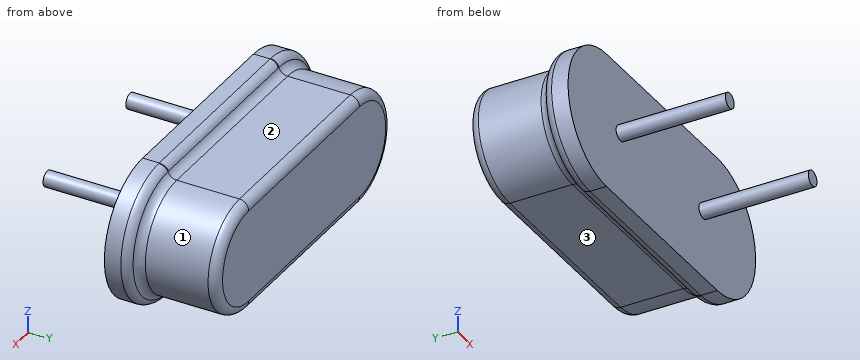
from build123d import *

# Parameters (mm, degrees)
SALIENTE_EXTRUIR1_DEPTH = 3.43
SALIENTE_EXTRUIR2_DEPTH = 0.8
REDONDEO2_R             = 0.3
REDONDEO5_R             = 0.3
CROQUIS2_R              = 0.25
SALIENTE_EXTRUIR3_DEPTH = 3.54


with BuildPart() as part:
    # Croquis1 → Saliente-Extruir1 (new body)
    with BuildSketch(Plane(origin=(0, 0, 0), x_dir=(1, 0, 0), z_dir=(0, 1, 0))):
        with BuildLine():
            Line((0, 0.4), (6.36, 0.4))
            ThreePointArc((6.36, 0.4), (8.16, 2.2), (6.36, 4))
            Line((6.36, 4), (0, 4))
            ThreePointArc((0, 4), (-1.8, 2.2), (0, 0.4))
        make_face()
    extrude(amount=SALIENTE_EXTRUIR1_DEPTH)

    # Croquis1_3 → Saliente-Extruir2 (add)
    with BuildSketch(Plane(origin=(0, 0, 0), x_dir=(1, 0, 0), z_dir=(0, 1, 0))):
        with BuildLine():
            Line((0, 0), (6.36, 0))
            ThreePointArc((6.36, 0), (8.56, 2.2), (6.36, 4.4))
            Line((6.36, 4.4), (0, 4.4))
            ThreePointArc((0, 4.4), (-2.2, 2.2), (0, 0))
        make_face()
        with BuildLine():
            Line((0, 0.4), (6.36, 0.4))
            ThreePointArc((6.36, 0.4), (8.16, 2.2), (6.36, 4))
            Line((6.36, 4), (0, 4))
            ThreePointArc((0, 4), (-1.8, 2.2), (0, 0.4))
        make_face(mode=Mode.SUBTRACT)
    extrude(amount=SALIENTE_EXTRUIR2_DEPTH)

    # Redondeo2
    redondeo2_edges = [part.edges().sort_by_distance(p)[0] for p in [
        (8.16, 3.43, -2.2),
        (3.18, 3.43, -4),
        (-1.8, 0.8, -2.2),
        (3.18, 0.8, -0.4),
        (8.16, 0.8, -2.2),
        (3.18, 0.8, -4),
        (-1.8, 3.43, -2.2),
        (3.18, 3.43, -0.4),
    ]]
    fillet(redondeo2_edges, radius=REDONDEO2_R)

    # Redondeo5
    redondeo5_edges = [part.edges().sort_by_distance(p)[0] for p in [
        (-2.2, 0.8, -2.2),
        (3.18, 0.8, -4.4),
        (8.56, 0.8, -2.2),
        (3.18, 0.8, 0),
    ]]
    fillet(redondeo5_edges, radius=REDONDEO5_R)

    # Croquis2 → Saliente-Extruir3 (add)
    with BuildSketch(Plane.XZ):
        with Locations(Location((0.805, -2.2, 0), (0, 0, 90))):
            Circle(CROQUIS2_R)
        with Locations(Location((5.555, -2.2, 0), (0, 0, 90))):
            Circle(CROQUIS2_R)
    extrude(amount=SALIENTE_EXTRUIR3_DEPTH)


solid = part.part
The listing builds one solid part. Answer for the finished solid, in the listing's coordinates (mm). Face numbers are marked on the shaded views. A direction names the side the tool comes from. Give positions to 0.01 mm unless a question says otherwise; leave off trailing zeros. Loops run counter-clockwise (first coordinate to the right, second up) from the corner with the lowest first, then second, coordinate; pieces in that order, holes last. Notation, with made-up numbers: (89, 3.25) - (141, 3.25) arc R37 ccw to (141, 40.25) - close; hole circle Ø5 at (-18.5, 45.25). An arc over 180 degrees is marked (long way). Use one line per item in the form item = value.
1. Find the intervals of material crossed by line 1 along Y through (x, z) = (7.25, -2.95); line 2 along X through (y, z) = (1.5, -1.2); line 3 along Z through (x, y) = (4.5, 3), in increasing order. Write a range as [from, to].
Calculated:
line_1 = [0, 3.43]
line_2 = [-1.5, 7.86]
line_3 = [-4, -0.4]
2. Which of the six approach directions +Z, -Z, +X, -X, +Y, -Y give full straight-line access (tool end or side, diameter ignored) to the marked faces 1, 2 and 3?
Calculated:
face_1 = +X, +Y
face_2 = +Z, +X, -X, +Y
face_3 = -Z, +X, -X, +Y
3. Section A-A on y = -1 is taken. Give the vertices of the cut face in (x, z) (3 decimals).
Calculated:
outline = circle Ø0.5 at (0.805, -2.2); circle Ø0.5 at (5.555, -2.2)
4. Section B-B on y = 1.25 is taken. Give the vertices of the cut face in (x, z).
Calculated:
outline = (0, -4) - (6.36, -4) arc R1.8 ccw to (6.36, -0.4) - (0, -0.4) arc R1.8 ccw to start
5. Given pin 1 Ø2 at (x, z) = (2.5, -2.5) entering from -Y; pin 2 Ø1.6 at (x, y) = (2, 2.5) entering from -Z; pin 3 Ø1 at (x, y) = (0.5, -2.5) entering from -Z, each flat-ended and moving along its own axis, determine where each tip first touches the part or whether it passes through.
Calculated:
pin_1 = 0
pin_2 = -4
pin_3 = -2.45
